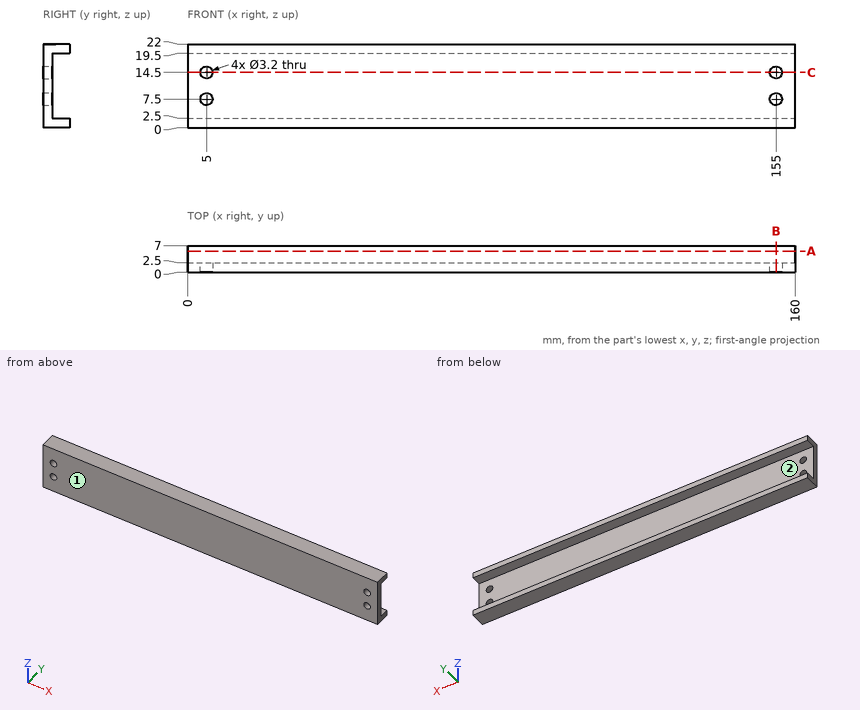
Source: three-view drawing plus pictorial views. Frame: mm from the lowest corner of the part. Round coordinates to 2 decimals unless told otherwise and drop trailing zeros. Loops run counter-clockwise (first coordinate to the right, second up) from the corner with the lowest first, then second, coordinate; pieces in that order, holes last. Notation, with made-up numbers: (28, 88) - (41, 88) arc R6 ccw to (41, 93) - close; hole circle Ø2 at (-15, 8.25). An arc over 180 degrees is marked (long way). Write each question's results on one line, items separated by ' | '. Start each with the question number.
1) Cut plane A-A on y = 5.5. Return loops of the section in (x, z).
2) Cut plane B-B on x = 155. Return loops of the section in (y, z), then the cut area to 3 significant figures.
3) Cut plane C-C on z = 14.5. Return loops of the section in (x, y).
4) Line query: probe 1 along X at (y, z) = (1.9, 7.5); probe 2 along Z at (x, y) = (155, 1); probe 3 along Z at (x, y) = (83.5, 3.5). Output: solid intervals per line, ascending. Write a range as [from, to].
5) First-contact query: P1, Ø6, axis at x = 55.5, z = 10, coming from the +Y side. Flat tip, straight axial feed; report the tip coordinate or a pass-through.
6) Mould query, pull axis Z, two halves, no side actions, for the marked faces 1 and 2. Classes: released by +Z, released by -Z, zero draft, split by the parting line, or undercut.
Verdict:
1) outline: (0, 0) - (160, 0) - (160, 2.5) - (0, 2.5) - close; (0, 19.5) - (160, 19.5) - (160, 22) - (0, 22) - close
2) outline: (0, 0) - (7, 0) - (7, 2.5) - (2.5, 2.5) - (2.5, 5.9) - (0, 5.9) - close; (0, 9.1) - (2.5, 9.1) - (2.5, 12.9) - (0, 12.9) - close; (0, 16.1) - (2.5, 16.1) - (2.5, 19.5) - (7, 19.5) - (7, 22) - (0, 22) - close | area: 61.5 mm2
3) outline: (0, 0) - (3.4, 0) - (3.4, 2.5) - (0, 2.5) - close; (6.6, 0) - (153.4, 0) - (153.4, 2.5) - (6.6, 2.5) - close; (156.6, 0) - (160, 0) - (160, 2.5) - (156.6, 2.5) - close
4) probe 1: x = [0, 3.4], [6.6, 153.4], [156.6, 160] | probe 2: z = [0, 5.9], [9.1, 12.9], [16.1, 22] | probe 3: z = [0, 2.5], [19.5, 22]
5) P1: stops at y = 2.5
6) face 1: zero draft | face 2: undercut
